Part model, mm, in its own coordinate system. A direction names the side the tool comes from. Round coordinates to 2 decimals unless told otherwise and drop trailing zeros. Write each loop counter-clockwise with the first axis right and the second up, starting at its lowest first coordinate (ties: lowest second). Pieces come first, ordered by that corner, then holes. Notation, with made-up numbers: (-8, 69) -> (17, 69) arc R19 ccw to (17, 84) -> close; hole circle Ø9 at (68.25, 37). An arc over 180 degrees is marked (long way). Return JSON: item names as keys, results as strings. Group by question number.
```python
from build123d import *

# Parameters (mm, degrees)
F1_DEPTH = 3
F2_D     = 6
F3_D     = 7
F4_D     = 6.1
F6_D     = 5
F7_D     = 8
F8_D     = 6


with BuildPart() as f1:
    # F0 (on Front) → F1 (new body)
    with BuildSketch(Plane.XZ):
        with BuildLine():
            Line((129, 0), (0, 0))
            Line((0, 0), (0, -105.5))
            Line((0, -105.5), (76, -105.5))
            ThreePointArc((76, -105.5), (79.1515590041, -106.6182895724), (80.8933757798, -109.4729296625))
            ThreePointArc((80.8933757798, -109.4729296625), (73.0885955883, -132.3000971657), (51, -142))
            Line((51, -142), (10, -142))
            Line((10, -142), (10, -154))
            Line((10, -154), (89, -154))
            Line((89, -154), (89, -138))
            Line((89, -138), (129, -138))
            Line((129, -138), (129, 0))
        make_face()
    extrude(amount=F1_DEPTH)

    # F2 (through all)
    with Locations(Plane(origin=(0, 0, 0), x_dir=(1, 0, 0), z_dir=(0, 1, 0))):
        with Locations((120, 5)):
            Hole(F2_D / 2)

    # F3 (through all)
    with Locations(Plane(origin=(0, 0, 0), x_dir=(1, 0, 0), z_dir=(0, 1, 0))):
        with Locations((15, 29), (31, 9), (105, 17.5)):
            Hole(F3_D / 2)

    # F4 (through all)
    with Locations(Plane(origin=(0, 0, 0), x_dir=(1, 0, 0), z_dir=(0, 1, 0))):
        with Locations((75, 72)):
            Hole(F4_D / 2)

    # F6 (through all)
    with Locations(Plane.XZ.offset(3)):
        with Locations((106.059, -89.975), (115, -91.3), (115, -82.3), (97.059, -89.975)):
            Hole(F6_D / 2)

    # F7 (through all)
    with Locations(Plane.XZ.offset(3)):
        with Locations((8.5, -71), (8.5, -54)):
            Hole(F7_D / 2)

    # F8 (through all)
    with Locations(Plane.XZ.offset(3)):
        with Locations((119.5, -108.667), (119.5, -126.667)):
            Hole(F8_D / 2)


solid = f1.part
```
Item 1: Wall check: L1, parallel to Z at x = 14.5, y = -1; L2, parallel to Z at x = 97, y = -2.1; L3, parallel to Z at x = 47.5, y = -0.65. Give the ranges that are in metal, low to high.
Item 2: Cut at D-D (z = -17.5). Write the cut outline in (x, y).
Item 3: Which spindle directions (+Z, -Z, +X, -X, +Y, -Y) get a long thin tool onto all of the face, cutting with end or side? Do faces 4 (the face through (79.114, -1.479, -106.588)), 5 (the face through (112.69, -1.48, -83.26)). Say none if no direction does.
Item 4: Cut at C-C (y = -1.15). State how many separate pieces and enclosed holes the cut face has, then the cut area to 3 significant figures.
Item 5: Cut at B-B (x = 15). Write the cut outline in (y, z).
Item 6: Cut at A-A (z = -82.3). Write the cut outline in (x, y), then the cut area to 3 significant figures.
Item 7: Flat gauge pins, fed straight in: P1, Ø1.5, axis at x = 106.5, y = -1, coming from the -Z side; P2, Ø5, axis at x = 120, z = -5, coming from the -Y side; P3, Ø1.5, axis at x = 44, z = -38.5, coming from the +Y side; P4, Ø0.9, axis at y = -1, z = -148.5, coming from the -X side. Where does each tip first touch, or does it go through?
Item 8: Two-plate mould, pull along X, no slides. Class faces 1 (the face through (116.73, -1.48, -127.82)), 2 (the face through (73.322, -1.479, -132.043)), 3 (the face through (64, -3, -59)): released by +X, released by -X, zero draft, split by the parting line, or undercut.
Checks:
{
 "1": {"L1": "z = -154 to -142, -105.5 to -32.46, -25.54 to 0", "L2": "z = -138 to -92.47, -87.48 to 0", "L3": "z = -154 to -142, -105.5 to 0"},
 "2": {"outline": "(0, -3) -> (101.5, -3) -> (101.5, 0) -> (0, 0) -> close; (108.5, -3) -> (129, -3) -> (129, 0) -> (108.5, 0) -> close"},
 "3": {"face 4": "-X, +Y, -Y", "face 5": "+Y, -Y"},
 "4": {"separate pieces": "1", "enclosed holes": "13", "area": "15,900 mm2"},
 "5": {"outline": "(-3, -154) -> (0, -154) -> (0, -142) -> (-3, -142) -> close; (-3, -105.5) -> (0, -105.5) -> (0, -32.5) -> (-3, -32.5) -> close; (-3, -25.5) -> (0, -25.5) -> (0, 0) -> (-3, 0) -> close"},
 "6": {"outline": "(0, -3) -> (112.5, -3) -> (112.5, 0) -> (0, 0) -> close; (117.5, -3) -> (129, -3) -> (129, 0) -> (117.5, 0) -> close", "area": "372 mm2"},
 "7": {"P1": "stops at z = -138", "P2": "passes through", "P3": "stops at y = 0", "P4": "stops at x = 10"},
 "8": {"face 1": "undercut", "face 2": "released by -X", "face 3": "zero draft"}
}
